Design review of the part built by this model. Coordinates are the model's own, in mm. Round coordinates to 2 decimals unless told otherwise and drop trailing zeros. Order: outer loops, then holes, each group sorted by start corner. A loop starts at its lowest first (then second) coordinate and runs counter-clockwise, first axis right, second up. Notation, with made-up numbers: M 65,43.25 L 101,43.25 A23 cw 101,79.25 Z; hole C 32,0.25 d7. An arc over 180 degrees is marked long. Write each question's results on one line, items separated by ' | '. Start each with the question number.
Item 1: Take a section at C-C, the plane z = 51.25. Write out the cut boundary in (x, y).
Item 2: Take a section at B-B, the plane y = -11. Write out the cut boundary in (x, z).
Item 3: The part is to be moulded in two halves that separate along X. For faces 1 (the flat face through (63, -55.499, 47)), 2 (the flat face through (0, -28, 45)), 3 (the flat face through (101.6, -54, 57)), 4 (the flat face through (25.4, -54, 57)), say which applies: +X half, -X half, draft (parallel to the pull), parting line (faces both ways), or undercut.
Item 4: Wall thickness on line 1 (X direction, y = -38, z = 59.75); line 2 (X direction, y = -30, z = 55.5); line 3 (Z direction, x = 102, y = -28): over which ranges is each line inside the solid? List them lowest first. Write a range as [from, to].
Item 5: Clearance check with flat-ended pins moving along their axes: pin 1 (2 mm diameter, centred on x = 61.5, z = 43.5, fed in from +Y); pin 2 (2 mm diameter, centred on y = -49, z = 56.5, fed in from +X). State where each tip first meets the part, or that it passes through.
```python
from build123d import *

# Parameters (mm, degrees)
F1_DEPTH = 127
F2_R     = 11.1125
F3_DEPTH = 6.35
F4_SIZE  = 0.254
F2_W     = 25.4
F2_H     = 3.175
F5_DEPTH = 1.778


with BuildPart() as f1:
    # F0 (on Right) → F1 (new body)
    with BuildSketch(Plane.YZ):
        Polygon((-55.499, 36.88551), (0, 36.88551), (0, 49.121089), (-55.499, 55.93551), align=None)
    extrude(amount=F1_DEPTH)

    # F2 (on face) → F3 (join)
    with BuildSketch(Plane(origin=(0, 5.941734, 48.391536), x_dir=(1, 0, 0), z_dir=(0, 0.121869, 0.992546))):
        with Locations((63.5, -44.439643)):
            Circle(F2_R)
    extrude(amount=F3_DEPTH)

    # F4
    f4_edges = [f1.edges().sort_by_distance(p)[0] for p in [
        (52.3875, -37.392792, 60.110034),
    ]]
    chamfer(f4_edges, length=F4_SIZE)

    # F2 (on face) → F5 (join)
    with BuildSketch(Plane(origin=(0, 5.941734, 48.391536), x_dir=(1, 0, 0), z_dir=(0, 0.121869, 0.992546))):
        with Locations((114.3, -60.314643)):
            Rectangle(F2_W, F2_H)
        with Locations((12.7, -60.314643)):
            Rectangle(F2_W, F2_H)
    extrude(amount=F5_DEPTH)


solid = f1.part
```
Results list:
1) outline: M 0,-55.5 L 127,-55.5 L 127,-17.34 L 0,-17.34 Z
2) outline: M 0,36.89 L 127,36.89 L 127,50.47 L 0,50.47 Z
3) face 1: draft | face 2: -X half | face 3: undercut | face 4: undercut
4) line 1: [52.4, 74.6] | line 2: [55.68, 71.32] | line 3: [36.89, 52.56]
5) pin 1: y = 0 | pin 2: x = 68.18
